Could you check a few things on this drawing? It's one solid part, dimensions in mm from its lowest x, y, z. Give positions to 0.01 mm unless a question says otherwise; leave off trailing zeros. Loops run counter-clockwise (first coordinate to the right, second up) from the corner with the lowest first, then second, coordinate; pieces in that order, holes last. Notation, with made-up numbers: (9.25, 46.5) -> (68.25, 46.5) arc R10 ccw to (68.25, 51.5) -> close; hole circle Ø6 at (-5.5, -31.75). An arc over 180 degrees is marked (long way). One line per question, with ' | ' between items.
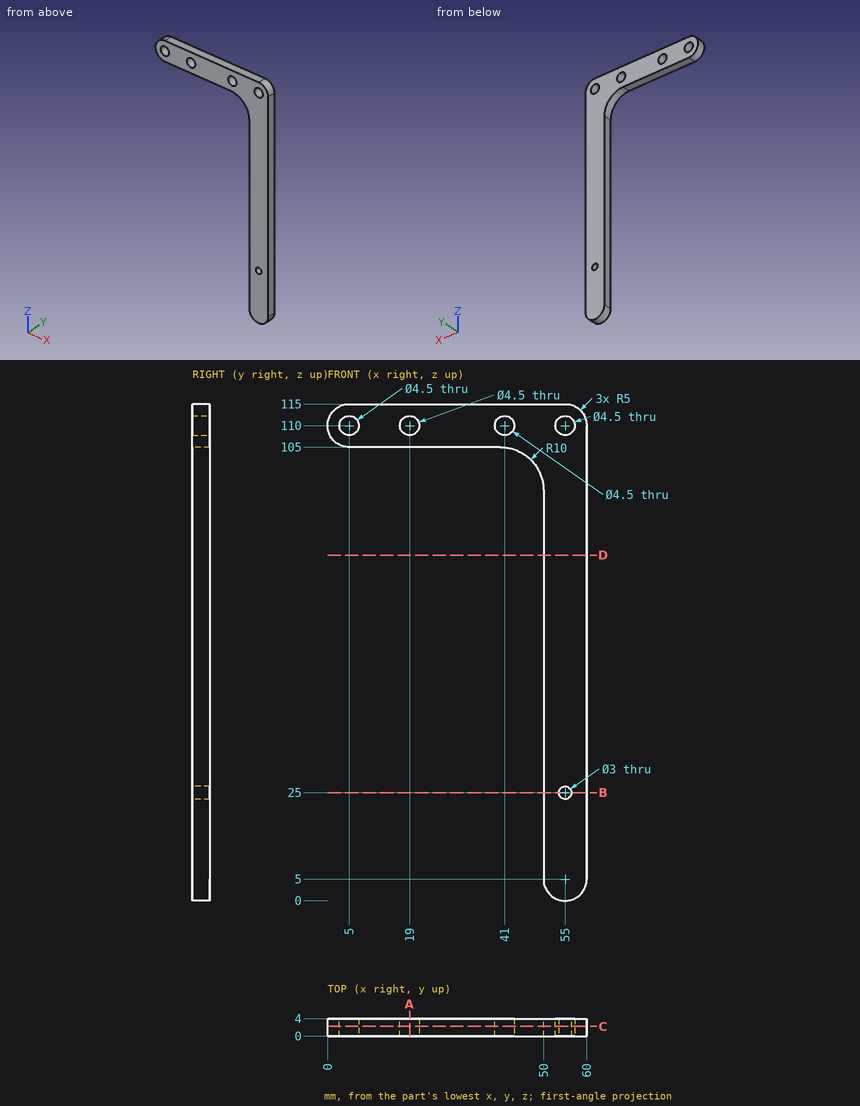
Q1. For pin 1 Ø2 at (y, z) = (2.5, 52.5) entering from -X; pin 2 Ø4 at (x, z) = (36, 102.5) entering from -Y, each with a flat end and sliding along its axis, tell me the tip position at first contact or that it passes through.
Entries:
pin 1: x = 50 | pin 2: through
Q2. If we section it at A-A (x = 19): Write out the boundary of the cut face in (y, z).
Entries:
outline: (0, 105) -> (4, 105) -> (4, 107.75) -> (0, 107.75) -> close; (0, 112.25) -> (4, 112.25) -> (4, 115) -> (0, 115) -> close
Q3. If we section it at D-D (z = 80): Write out the boundary of the cut face in (x, y), plus the area to 3 significant figures.
Entries:
outline: (50, 0) -> (60, 0) -> (60, 4) -> (50, 4) -> close | area: 40.0 mm²
Q4. If we section it at B-B (z = 25): Write out the boundary of the cut face in (x, y), plus the area to 3 significant figures.
Entries:
outline: (50, 0) -> (53.5, 0) -> (53.5, 4) -> (50, 4) -> close; (56.5, 0) -> (60, 0) -> (60, 4) -> (56.5, 4) -> close | area: 28.0 mm²
Q5. If I drill on probe 1 along Z at (x, y) = (55, 1.7); probe 2 along X at (y, z) = (2.9, 110); probe 3 along Z at (x, y) = (5, 2.2), over which ranges is the centre line in solid material (lowest first)? Write a range as from..to.
Entries:
probe 1: 0..23.5, 26.5..107.75, 112.25..115 | probe 2: 0..2.75, 7.25..16.75, 21.25..38.75, 43.25..52.75, 57.25..60 | probe 3: 105..107.75, 112.25..115
Q6. If we section it at C-C (y = 2.2): Write out the boundary of the cut face in (x, z).
Entries:
outline: (5, 105) -> (40, 105) arc R10 cw to (50, 95) -> (50, 5) arc R5 ccw to (60, 5) -> (60, 110) arc R5 ccw to (55, 115) -> (5, 115) arc R5 ccw to start; hole circle Ø4.5 at (5, 110); hole circle Ø4.5 at (19, 110); hole circle Ø4.5 at (41, 110); hole circle Ø4.5 at (55, 110); hole circle Ø3 at (55, 25)
